Part model, mm, in its own coordinate system. A direction names the side the tool comes from. Round coordinates to 2 decimals unless told otherwise and drop trailing zeros. Write each loop counter-clockwise with the first axis right and the second up, starting at its lowest first coordinate (ties: lowest second). Pieces come first, ordered by that corner, then holes. Notation, with made-up numbers: M 55,-28.5 L 88,-28.5 A21 cw 88,-18.5 Z; hole C 52,-25.5 d10. An arc over 180 degrees is marked long. One line per question, with ' | ' between items. Start each with the question number.
1) Saw through at C-C (x = -8.5). List the corners of the cut face in (y, z).
2) Wall check: probe 1 along Y at (x, z) = (-3, 5.5); probe 2 along Y at (x, z) = (13.5, 7.5); probe 3 along X at (y, z) = (-6.5, 6). Give the ranges that are in metal, low to high. Write a range as [from, to].
3) Saw through at A-A (x = 13). List the corners of the cut face in (y, z), plus the area to 3 significant figures.
4) Tool access for faces 1 (the face through (-13.196, -1.691, 9.136)), 2 (the face through (1.01, -3.85, -0.44)): list every direction of +Z, -Z, +X, -X, +Y, -Y with a clear straight run to the whole face (end or side of a thin tool).
5) Mould opens along Y. For faces 3 (the face through (4, -2.555, 0)), 4 (the face through (-13.21, -1.69, -9.12)), 5 (the face through (3, 13, 10.222)) say: pulls with the +Y half, pulls with the -Y half, needs draft (parallel to the pull), parting line crosses it, or undercut.
6) Saw through at D-D (z = 0). List the corners of the cut face in (x, y), plus the area to 3 significant figures.
7) Saw through at B-B (z = 7). List the corners of the cut face in (x, y).
```python
from build123d import *

# Parameters (mm, degrees)
SKETCH_1_R      = 5
EXTRUDE_1_DEPTH = 2
SKETCH_2_R      = 2
EXTRUDE_2_DEPTH = 1.5
EXTRUDE_3_DEPTH = 18
FILLET_1_R      = 1
CHAMFER_1_SIZE  = 1
SCALE_1_SCALE   = 1.703703703


with BuildPart() as part:
    # 草图1 → 凸台-拉伸1 (new body)
    with BuildSketch(Plane(origin=(0, 0, 0), x_dir=(1, 0, 0), z_dir=(0, 1, 0))):
        with Locations(Location((0, 0, 0), (0, 0, 270))):
            Circle(SKETCH_1_R)
    extrude(amount=EXTRUDE_1_DEPTH)

    # 草图2 → 凸台-拉伸2 (add)
    with BuildSketch(Plane(origin=(0, 2, 0), x_dir=(1, 0, 0), z_dir=(0, 1, 0))):
        with Locations(Location((0, 0, 0), (0, 0, 270))):
            Circle(SKETCH_2_R)
    extrude(amount=EXTRUDE_2_DEPTH)

    # 草图3 → 凸台-拉伸3 (add)
    with BuildSketch(Plane(origin=(0, 3.5, 0), x_dir=(1, 0, 0), z_dir=(0, 1, 0))):
        Polygon((0, -6), (-7, -6), (-7, 6), (0, 6), (14, 6), (14, -6), align=None)
    extrude(amount=EXTRUDE_3_DEPTH)

    # 圆角1
    fillet_1_edges = [part.edges().sort_by_distance(p)[0] for p in [
        (14, 12.5, 6),
        (14, 12.5, -6),
        (-7, 12.5, -6),
        (-7, 12.5, 6),
        (3.5, 21.5, 6),
        (14, 21.5, 0),
        (3.5, 21.5, -6),
        (-7, 21.5, 0),
    ]]
    fillet(fillet_1_edges, radius=FILLET_1_R)

    # 倒角1
    chamfer_1_edges = [part.edges().sort_by_distance(p)[0] for p in [
        (-7, 3.5, 0),
        (3.5, 3.5, -6),
        (14, 3.5, 0),
        (3.5, 3.5, 6),
        (-6.707106781, 3.5, -5.707106781),
        (-6.707106781, 3.5, 5.707106781),
        (13.707106781, 3.5, -5.707106781),
        (13.707106781, 3.5, 5.707106781),
    ]]
    chamfer(chamfer_1_edges, length=CHAMFER_1_SIZE)


with BuildPart() as part_1:
    # 缩放比例1: scaled about (3.367633963, 12.104632395, 0)
    add(part.part.scale(SCALE_1_SCALE).moved(Location((-2.36981649, -8.518074639, 0))))


solid = part_1.part
```
Answer key:
1) outline: M -8.52,-5.91 L -5.11,-5.91 L -5.11,5.91 L -8.52,5.91 Z; M -2.56,-8.52 L -0.85,-10.22 L 26.41,-10.22 A1.7 ccw 28.11,-8.52 L 28.11,8.52 A1.7 ccw 26.41,10.22 L -0.85,10.22 L -2.56,8.52 Z
2) probe 1: y = [-8.52, -5.11], [-2.56, 28.11] | probe 2: y = [-2.56, 28.11] | probe 3: x = [-8.42, 3.68]
3) outline: M -2.56,-8.52 L -0.85,-10.22 L 26.41,-10.22 A1.7 ccw 28.11,-8.52 L 28.11,8.52 A1.7 ccw 26.41,10.22 L -0.85,10.22 L -2.56,8.52 Z | area: 623 mm2
4) face 1: +Z, -X, -Y | face 2: none
5) face 3: undercut | face 4: pulls with the -Y half | face 5: needs draft
6) outline: M -14.3,-0.85 L -12.59,-2.56 L -5.78,-2.56 L -5.78,-5.11 L -10.89,-5.11 L -10.89,-8.52 L 6.15,-8.52 L 6.15,-5.11 L 1.04,-5.11 L 1.04,-2.56 L 19.78,-2.56 L 21.48,-0.85 L 21.48,26.41 A1.7 ccw 19.78,28.11 L -12.59,28.11 A1.7 ccw -14.3,26.41 Z | area: 1,170 mm2
7) outline: M -14.3,-0.85 L -12.59,-2.56 L 19.78,-2.56 L 21.48,-0.85 L 21.48,26.41 A1.7 ccw 19.78,28.11 L -12.59,28.11 A1.7 ccw -14.3,26.41 Z; M -7.22,-8.52 L 2.48,-8.52 L 2.48,-5.11 L -7.22,-5.11 Z
